Model file for the job. Use its own axes, mm. Round coordinates to 2 decimals unless told otherwise and drop trailing zeros. Order: outer loops, then holes, each group sorted by start corner. A loop starts at its lowest first (then second) coordinate and runs counter-clockwise, first axis right, second up. Notation, with made-up numbers: (63.25, -1) - (80.25, -1) arc R18 ccw to (80.25, 28) - close; hole circle Ø11 at (-32, 61). An arc over 180 degrees is marked (long way). Use one line per item in the form item = value.
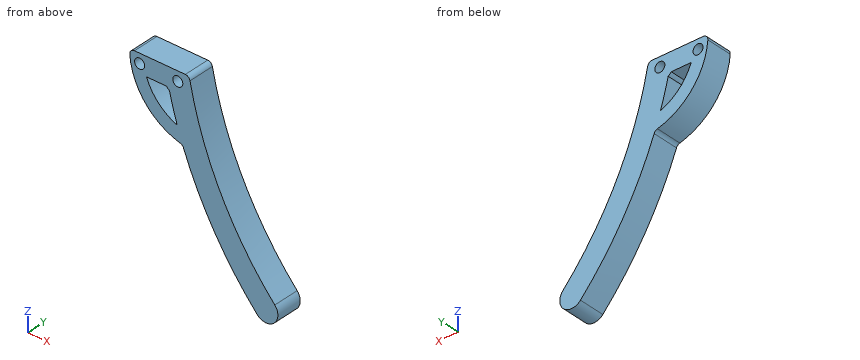
from build123d import *

# Parameters (mm, degrees)
SKETCH1_R           = 2.1
BOSS_EXTRUDE1_DEPTH = 11
FILLET1_R           = 2


with BuildPart() as part:
    # Sketch1 → Boss-Extrude1 (new body)
    with BuildSketch(Plane(origin=(0, 0, 0), x_dir=(1, 0, 0), z_dir=(0, 1, 0))):
        with BuildLine():
            Line((-169.316682473, 27), (-144.285495113, 27))
            ThreePointArc((-144.285495113, 27), (-131.38096704, 65.470188633), (-108.437297629, 98.937639869))
            ThreePointArc((-108.437297629, 98.937639869), (-108.760877497, 106.001300115), (-115.824537743, 105.677720247))
            ThreePointArc((-115.824537743, 105.677720247), (-133.944213048, 81.498784597), (-147.089597617, 54.293225847))
            ThreePointArc((-147.089597617, 54.293225847), (-163.056941322, 44.599456514), (-169.316682473, 27))
        make_face()
        with Locations(Location((-149.101129521, 31, 0), (0, 0, 270))):
            Circle(SKETCH1_R, mode=Mode.SUBTRACT)
        with Locations(Location((-165.101129521, 31, 0), (0, 0, 270))):
            Circle(SKETCH1_R, mode=Mode.SUBTRACT)
        with BuildLine():
            Line((-162.242742421, 34.797226479), (-153.870589387, 34.797226479))
            ThreePointArc((-153.870589387, 34.797226479), (-153.279814844, 35.43906131), (-152.603484102, 35.990008892))
            ThreePointArc((-152.603484102, 35.990008892), (-151.085722301, 41.907142789), (-149.338618997, 47.76066348))
            ThreePointArc((-149.338618997, 47.76066348), (-157.187118972, 42.668993907), (-162.242742421, 34.797226479))
        make_face(mode=Mode.SUBTRACT)
    extrude(amount=BOSS_EXTRUDE1_DEPTH)

    # Fillet1
    fillet1_edges = [part.edges().sort_by_distance(p)[0] for p in [
        (-147.089597617, 5.5, -54.293225847),
        (-144.285495113, 5.5, -27),
        (-169.316682473, 5.5, -27),
    ]]
    fillet(fillet1_edges, radius=FILLET1_R)


solid = part.part
(1) Slice it at B-B on z = -31. Give the cut face in (x, y).
Report:
outline = (-169.03, 0) - (-167.2, 0) - (-167.2, 11) - (-169.03, 11) - close; (-163, 0) - (-151.2, 0) - (-151.2, 11) - (-163, 11) - close; (-147, 0) - (-143.48, 0) - (-143.48, 11) - (-147, 11) - close
(2) Pin check, flat tips, straight feed: pin 1 (3 mm diameter, centred on y = 3.5, z = -59, fed in from -X); pin 2 (5 mm diameter, centred on y = 3.5, z = -74, fed in from +X); pin 3 (2.5 mm diameter, centred on x = -159, y = 7.5, fed in from -Z). Stop position of each tip, or through.
Report:
pin_1 = -145.87
pin_2 = -125.28
pin_3 = -49.6
(3) Slice it at A-A on z = -44.5. Give the cut face in (x, y).
Report:
outline = (-163.14, 0) - (-155.12, 0) - (-155.12, 11) - (-163.14, 11) - close; (-150.34, 0) - (-139.88, 0) - (-139.88, 11) - (-150.34, 11) - close
(4) Slice it at D-D on y = 5.75. Count the separate pieces of the cut face and the enclosed holes in it, then the cut area to 3 significant figures.
Report:
separate_pieces = 1
enclosed_holes = 3
area = 1,120 mm2
(5) Slice it at C-C on x = -114. Give the cut face in (y, z).
Report:
outline = (0, -106.95) - (11, -106.95) - (11, -92.47) - (0, -92.47) - close
(6) Probe probe 1 along X at (y, z) = (2.5, -31); probe 2 along X at (y, z) = (6, -42); probe 3 along X at (y, z) = (4.5, -44). List the from-to ranges inside material, lowest first. Write a range as [from, to].
Report:
probe_1 = [-169.03, -167.2], [-163, -151.2], [-147, -143.48]
probe_2 = [-164.94, -157.83], [-151.06, -140.65]
probe_3 = [-163.53, -155.74], [-150.49, -140.04]
